Here's how the part is built. I have some questions about the finished solid (model axes, mm). A direction names the side the tool comes from. Give positions to 0.01 mm unless a question says otherwise; leave off trailing zeros. Write each loop counter-clockwise with the first axis right and the second up, starting at its lowest first coordinate (ties: lowest second). Pieces come first, ordered by that corner, then holes. Notation, with made-up numbers: (1.25, -25.75) - (11.25, -25.75) arc R27 cw to (11.25, 5.25) - close; hole circle Ø9 at (63.5, -4). An arc over 180 degrees is marked (long way). One line per item, written item: value. Start each with the question number.
1) I'm going to push flat-ended pins straight in: P1, Ø6.5, axis at x = -70.5, z = 23.5, coming from the +Y side; P2, Ø9, axis at x = 0, y = 83, coming from the +Z side; P3, Ø5, axis at x = 71, z = 24, coming from the +Y side; P4, Ø1.8, axis at x = -71, z = 24, coming from the +Y side. Where does each tip first touch, or does it pass through?
2) On a 3-axis mill with a long thin cutter (end or side, diameter ignored), from which of +Z, -Z, +X, -X, +Y, -Y can I reach the whole of each face in a straight line? I mean faces 1 (the flat face through (65, 48, 23)), 2 (the flat face through (72.3, 56, 22.7)). Say none if no direction works.
3) Imagine slicing it at B-B on x = 0. Write out the boundary of the cut face in (y, z), plus the area to 3 significant figures.
4) Imagine slicing it at C-C on y = 72. Write out the boundary of the cut face in (x, z), plus the area to 3 significant figures.
5) We'd pull the mould along Z, two halves only. Please class faces 3 (the flat face through (-69.7, 56, 22.7)), 4 (the flat face through (0, 82, 25)), 5 (the cylindrical face through (0, 75, 28)), 6 (the flat face through (-1, 76, 16)): +Z half, -Z half, draft (parallel to the pull), parting line (faces both ways), or undercut.
6) Imagine slicing it at A-A on y = 51.5. Write out the boundary of the cut face in (x, z).
7) Please list where these lines run through material, in increasing order: L1, parallel to Z at x = 71, y = 52; L2, parallel to Z at x = 71, y = 58; L3, parallel to X at y = 51, z = 24. Write a range as [from, to].
8) Imagine slicing it at D-D on x = 71. Write out the boundary of the cut face in (y, z).
from build123d import *

# Parameters (mm, degrees)
CYLINDER684_R     = 8
CYLINDER684_DEPTH = 6
CYLINDER677_R     = 3
CYLINDER677_DEPTH = 50
CYLINDER678_R     = 3
CYLINDER678_DEPTH = 50
CYLINDER670_R     = 1.5
CYLINDER670_DEPTH = 50
CYLINDER679_R     = 1.5
CYLINDER679_DEPTH = 50
CYLINDER667_R     = 74
CYLINDER667_DEPTH = 15
CYLINDER665_R     = 46
CYLINDER665_DEPTH = 36
CYLINDER666_R     = 46
CYLINDER666_DEPTH = 36
BOX752_W          = 148
BOX752_H          = 38
BOX752_DEPTH      = 15


with BuildPart() as obj1:
    # Cylinder684 → Cylinder684 (new body)
    with BuildSketch(Plane(origin=(0, 83, 25), x_dir=(1, 0, 0), z_dir=(0, 0, 1))):
        Circle(CYLINDER684_R)
    extrude(amount=CYLINDER684_DEPTH)


with BuildPart() as obj2:
    # Cylinder677 → Cylinder677 (new body)
    with BuildSketch(Plane(origin=(-71, 106, 24), x_dir=(1, 0, 0), z_dir=(0, -1, 0))):
        Circle(CYLINDER677_R)
    extrude(amount=CYLINDER677_DEPTH)


with BuildPart() as compound398:
    # Cylinder678 → Cylinder678 (new body)
    with BuildSketch(Plane(origin=(71, 106, 24), x_dir=(1, 0, 0), z_dir=(0, -1, 0))):
        Circle(CYLINDER678_R)
    extrude(amount=CYLINDER678_DEPTH)

    # Compound398: union obj2
    add(obj2.part)


with BuildPart() as obj3:
    # Cylinder670 → Cylinder670 (new body)
    with BuildSketch(Plane(origin=(-71, 80, 24), x_dir=(1, 0, 0), z_dir=(0, -1, 0))):
        Circle(CYLINDER670_R)
    extrude(amount=CYLINDER670_DEPTH)


with BuildPart() as compound395:
    # Cylinder679 → Cylinder679 (new body)
    with BuildSketch(Plane(origin=(71, 80, 24), x_dir=(1, 0, 0), z_dir=(0, -1, 0))):
        Circle(CYLINDER679_R)
    extrude(amount=CYLINDER679_DEPTH)

    # Compound395: union obj3
    add(obj3.part)


with BuildPart() as obj4:
    # Cylinder667 → Cylinder667 (new body)
    with BuildSketch(Plane.XY.offset(16)):
        Circle(CYLINDER667_R)
    extrude(amount=CYLINDER667_DEPTH)


with BuildPart() as obj5:
    # Cylinder665 → Cylinder665 (new body)
    with BuildSketch(Plane(origin=(76.3, 104, 16), x_dir=(1, 0, 0), z_dir=(0, 0, 1))):
        Circle(CYLINDER665_R)
    extrude(amount=CYLINDER665_DEPTH)


with BuildPart() as obj6:
    # Cylinder666 → Cylinder666 (new body)
    with BuildSketch(Plane(origin=(-76.3, 104, 16), x_dir=(1, 0, 0), z_dir=(0, 0, 1))):
        Circle(CYLINDER666_R)
    extrude(amount=CYLINDER666_DEPTH)


with BuildPart() as cut278:
    # Box752 → Box752 (new body)
    with BuildSketch(Plane(origin=(-74, 48, 16), x_dir=(1, 0, 0), z_dir=(0, 0, 1))):
        with Locations((74, 19)):
            Rectangle(BOX752_W, BOX752_H)
    extrude(amount=BOX752_DEPTH)

    # Cut269: cut obj6
    add(obj6.part, mode=Mode.SUBTRACT)

    # Cut270: cut obj5
    add(obj5.part, mode=Mode.SUBTRACT)

    # Cut267: cut obj4
    add(obj4.part, mode=Mode.SUBTRACT)

    # Cut272: cut Compound395
    add(compound395.part, mode=Mode.SUBTRACT)

    # Cut273: cut Compound398
    add(compound398.part, mode=Mode.SUBTRACT)

    # Cut278: cut obj1
    add(obj1.part, mode=Mode.SUBTRACT)


solid = cut278.part
Numbers:
1. P1: y = 58.9
1. P2: z = 25
1. P3: y = 56
1. P4: through
2. face 1: +Z, -Z, +X, -X, -Y
2. face 2: +Y
3. outline: (74, 16) - (86, 16) - (86, 25) - (75, 25) - (75, 31) - (74, 31) - close
3. area: 114 mm^2
4. outline: (-43.25, 16) - (-17.09, 16) - (-17.09, 31) - (-43.25, 31) - close; (17.09, 16) - (43.25, 16) - (43.25, 31) - (17.09, 31) - close
4. area: 785 mm^2
5. face 3: undercut
5. face 4: +Z half
5. face 5: draft
5. face 6: -Z half
6. outline: (-74, 16) - (-53.14, 16) - (-53.14, 31) - (-74, 31) - close; (53.14, 16) - (74, 16) - (74, 31) - (53.14, 31) - close; hole circle Ø3 at (-71, 24); hole circle Ø3 at (71, 24)
7. L1: [16, 22.5], [25.5, 31]
7. L2: [16, 21], [27, 31]
7. L3: [-74, -72.5], [-69.5, -53.62], [53.62, 69.5], [72.5, 74]
8. outline: (48, 16) - (58.31, 16) - (58.31, 21) - (56, 21) - (56, 22.5) - (48, 22.5) - close; (48, 25.5) - (56, 25.5) - (56, 27) - (58.31, 27) - (58.31, 31) - (48, 31) - close
